Verification items for this drawing (mm, ordinates from the low corner). A direction names the side the tool comes from. Give positions to 0.01 mm unless a question says otherwise; leave off trailing zeros. Write each loop counter-clockwise with the first axis right and the second up, starting at its lowest first coordinate (ties: lowest second). Pieces come first, ordered by that corner, then holes. Notation, with made-up numbers: (4.25, 28) -> (41.25, 28) arc R22 cw to (41.25, 46) -> close; hole circle Ø4 at (54, 10.5). An arc over 180 degrees is marked (long way). Answer as a JSON object with one key per item and string values.
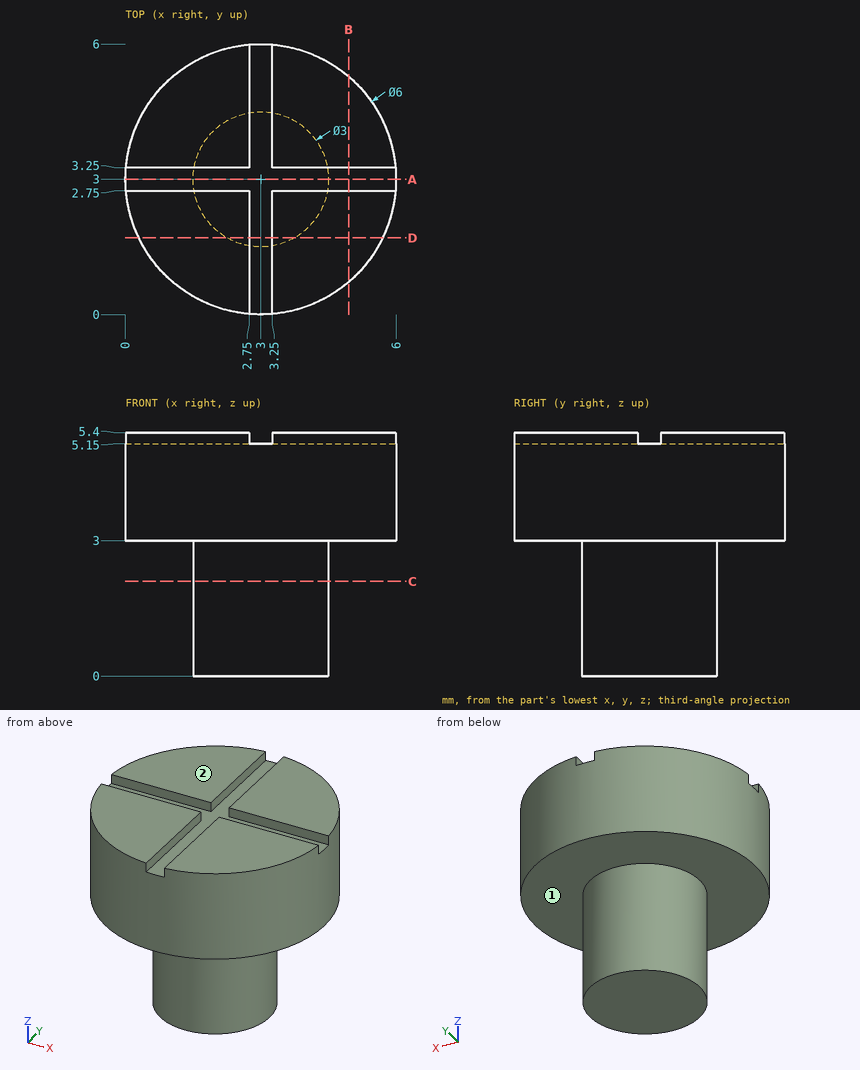
1. Sectioned sample at D-D, the plane y = 1.7. Enter the section's corners in (x, z), plus the area to 3 significant figures.
Determined:
{"outline": "(0.3, 3) -> (2.25, 3) -> (2.25, 0) -> (3.75, 0) -> (3.75, 3) -> (5.7, 3) -> (5.7, 5.4) -> (3.25, 5.4) -> (3.25, 5.15) -> (2.75, 5.15) -> (2.75, 5.4) -> (0.3, 5.4) -> close", "area": "17.3 mm^2"}
2. Go/stop test with flat-tipped pins: P1, Ø1.8, axis at x = 3.5, y = 3, coming from the +Z side; P2, Ø3, axis at y = 2.5, z = 1, coming from the +X side; P3, Ø1.5, axis at y = 0.5, z = 4.5, coming from the -X side; P4, Ø2, axis at x = 2, z = 2.5, coming from the +Y side. Record where each tip stops, or that it passes through.
Determined:
{"P1": "z = 5.4", "P2": "x = 4.5", "P3": "x = 0.56", "P4": "y = 6"}
3. Sectioned sample at B-B, the plane x = 4.95. Enter the section's corners in (y, z), plus the area to 3 significant figures.
Determined:
{"outline": "(0.72, 3) -> (5.28, 3) -> (5.28, 5.4) -> (3.25, 5.4) -> (3.25, 5.15) -> (2.75, 5.15) -> (2.75, 5.4) -> (0.72, 5.4) -> close", "area": "10.8 mm^2"}
4. Scan lines: L1, parallel to Z at x = 3.5, y = 3; L2, parallel to Z at x = 5, y = 2.4; L3, parallel to Y at x = 2.95, z = 1. Record each from-to range of solid material in increasing order. Write a range as [from, to].
Determined:
{"L1": "[0, 5.15]", "L2": "[3, 5.4]", "L3": "[1.5, 4.5]"}
5. Sectioned sample at A-A, the plane y = 3. Enter the section's corners in (x, z), plus the area to 3 significant figures.
Determined:
{"outline": "(0, 3) -> (1.5, 3) -> (1.5, 0) -> (4.5, 0) -> (4.5, 3) -> (6, 3) -> (6, 5.15) -> (0, 5.15) -> close", "area": "21.9 mm^2"}
6. Sectioned sample at C-C, the plane z = 2.1. Enter the section's corners in (x, y).
Determined:
{"outline": "circle Ø3 at (3, 3)"}
7. Access from +Z, -Z, +X, -X, +Y, -Y to the whole of each face (thin tool, end or side, straight path). Record for the marked faces 1 and 2.
Determined:
{"face 1": "-Z", "face 2": "+Z, +X, -X, +Y, -Y"}
